The model under review builds one solid part; all positions refer to its coordinate system, in mm. A direction names the side the tool comes from. Round coordinates to 2 decimals unless told otherwise and drop trailing zeros. Order: outer loops, then holes, each group sorted by start corner. A loop starts at its lowest first (then second) coordinate and runs counter-clockwise, first axis right, second up.
Solid Edge part; units mm, degrees
sketch "Sketch1" plane through (0, 0, 0) normal (1, 0, 0) x (0, 1, 0)
  line L0 (3, 0) -> (3, 20)
  line L1 (3, 20) -> (23, 20)
  line L2 (23, 20) -> (14.7157, 0)
  line L3 (14.7157, 0) -> (3, 0)
  dimension "D1" = 3
  dimension "D2" = 3
  dimension "D3" = 14.7157
revolve "RevolvedProtrusion1" add sketch "Sketch1" angle 360 about axis through (0, 0, 0) along (0, 0, 1)
sketch "Sketch2" plane through (0, 0, 20) normal (0, 0, 1) x (1, 0, 0)
  circle A0 centre (0, 0) radius 7.5
  line L0 (1.5, 8.5) -> (-1.5, 8.5)
  line L1 (-1.5, 8.5) -> (-1.5, 6.5)
  line L2 (-1.5, 6.5) -> (1.5, 6.5)
  line L3 (1.5, 6.5) -> (1.5, 8.5)
extrude "Cutout1" cut sketch "Sketch2" against normal up to surface (20 mm away)
fillet "Round1" radius 1 2 edges at (-23, 0, 20) (-14.7157, 0, 0)
(1) Tool access review of faces 4 (the flat face through (-1.5, 8, 10)), 5 (the flat face through (0, 9, 20)): name each direction out of +Z, -Z, +X, -X, +Y, -Y from which nothing blocks a thin tool from reaching the whole face with its end or side.
(2) We need section C-C (z = 13.5). Give the boundary of the cut face in (x, y).
(3) Clearance check with flat-ended pins moving along their axes: P1, Ø1.5, axis at y = -3.5, z = 12.5, coming from the +X side; P2, Ø8, axis at y = -7.5, z = 11.5, coming from the +X side; P3, Ø0.6, axis at y = 7.5, z = 7, coming from the +X side. State where each tip first meets the part, or that it passes through.
(4) We need section A-A (x = 0). Give the boundary of the cut face in (y, z).
(5) We need section D-D (z = 5.25). Give the boundary of the cut face in (x, y), and give its area (3 significant figures).
(6) We need section B-B (y = 0). Give the boundary of the cut face in (x, z), and give its area (3 significant figures).
(7) The part is to be moulded in two halves that separate along Y. For faces 1 (the flat face through (1.5, 8, 10)), 2 (the flat face through (6, 6, 0)), 3 (the conical face through (15.879, -3.526, 3.743)), say which applies: pulls with the +Y half, pulls with the -Y half, needs draft (parallel to the pull), parting line crosses it, or undercut.
(8) To check wall thickness, follow L1, parallel to X at y = 0, z = 7.5; L2, parallel to X at y = -4, z = 10.5; L3, parallel to Y at x = -2, z = 4.25. State the ranges of each line that lie inside material, in increasing order.
Verdict:
1. face 4: +Z, -Z
1. face 5: +Z, +X, -X, +Y, -Y
2. outline: circle Ø40.62 at (0, 0); hole (-1.5, 7.35) arc R7.5 ccw (long way) to (1.5, 7.35) - (1.5, 8.5) - (-1.5, 8.5) - close
3. P1: stops at x = 19.92
3. P2: stops at x = 20.18
3. P3: stops at x = 16.13
4. outline: (-22.43, 18.62) - (-14.97, 0.62) arc R1 ccw to (-14.05, 0) - (-7.5, 0) - (-7.5, 20) - (-21.5, 20) arc R1 ccw to start; (8.5, 0) - (14.05, 0) arc R1 ccw to (14.97, 0.62) - (22.43, 18.62) arc R1 ccw to (21.5, 20) - (8.5, 20) - close
5. outline: circle Ø33.78 at (0, 0); hole (-1.5, 7.35) arc R7.5 ccw (long way) to (1.5, 7.35) - (1.5, 8.5) - (-1.5, 8.5) - close
5. area: 716 mm2
6. outline: (-22.43, 18.62) - (-14.97, 0.62) arc R1 ccw to (-14.05, 0) - (-7.5, 0) - (-7.5, 20) - (-21.5, 20) arc R1 ccw to start; (7.5, 0) - (14.05, 0) arc R1 ccw to (14.97, 0.62) - (22.43, 18.62) arc R1 ccw to (21.5, 20) - (7.5, 20) - close
6. area: 453 mm2
7. face 1: undercut
7. face 2: needs draft
7. face 3: parting line crosses it
8. L1: x = -17.82 to -7.5, 7.5 to 17.82
8. L2: x = -18.64 to -6.34, 6.34 to 18.64
8. L3: y = -16.35 to -7.23, 7.23 to 16.35
